from build123d import *

# Parameters (mm, degrees)
SKETCH1_W           = 23
SKETCH1_H           = 37.5
BOSS_EXTRUDE1_DEPTH = 48.5
SKETCH2_W           = 12.6
SKETCH2_H           = 24
CUT_EXTRUDE1_DEPTH  = 43.5
SKETCH3_W           = 12.6
SKETCH3_H           = 3
CUT_EXTRUDE2_DEPTH  = 5
SKETCH4_W           = 10
SKETCH4_H           = 2
BOSS_EXTRUDE2_DEPTH = 10
SKETCH5_W           = 10
SKETCH5_H           = 2
BOSS_EXTRUDE3_DEPTH = 10
SKETCH6_R           = 1.5
CUT_EXTRUDE3_DEPTH  = 10


with BuildPart() as part:
    # Sketch1 → Boss-Extrude1 (new body)
    with BuildSketch(Plane(origin=(0, 0, 0), x_dir=(1, 0, 0), z_dir=(0, 1, 0))):
        Rectangle(SKETCH1_W, SKETCH1_H)
    extrude(amount=BOSS_EXTRUDE1_DEPTH)

    # Sketch2 → Cut-Extrude1 (cut)
    with BuildSketch(Plane(origin=(0, 48.5, 0), x_dir=(1, 0, 0), z_dir=(0, 1, 0))):
        with Locations((0, -6.75)):
            Rectangle(SKETCH2_W, SKETCH2_H)
    extrude(amount=-CUT_EXTRUDE1_DEPTH, mode=Mode.SUBTRACT)

    # Sketch3 → Cut-Extrude2 (cut)
    with BuildSketch(Plane.XY.offset(-5.25)):
        with Locations((0, 26.5)):
            Rectangle(SKETCH3_W, SKETCH3_H)
    extrude(amount=-CUT_EXTRUDE2_DEPTH, mode=Mode.SUBTRACT)

    # Sketch4 → Boss-Extrude2 (add)
    with BuildSketch(Plane.ZY.offset(11.5)):
        with Locations((-13.75, 47.5)):
            Rectangle(SKETCH4_W, SKETCH4_H)
    extrude(amount=BOSS_EXTRUDE2_DEPTH)

    # Sketch5 → Boss-Extrude3 (add)
    with BuildSketch(Plane(origin=(11.5, 0, 0), x_dir=(0, 0, -1), z_dir=(1, 0, 0))):
        with Locations((13.75, 47.5)):
            Rectangle(SKETCH5_W, SKETCH5_H)
    extrude(amount=BOSS_EXTRUDE3_DEPTH)

    # Sketch6 → Cut-Extrude3 (cut)
    with BuildSketch(Plane(origin=(0, 48.5, 0), x_dir=(1, 0, 0), z_dir=(0, 1, 0))):
        with Locations(Location((16.5, 13.75, 0), (0, 0, 270))):
            Circle(SKETCH6_R)
        with Locations(Location((-16.5, 13.75, 0), (0, 0, 270))):
            Circle(SKETCH6_R)
    extrude(amount=-CUT_EXTRUDE3_DEPTH, mode=Mode.SUBTRACT)


solid = part.part
Model file for the job. Use its own axes, mm. A direction names the side the tool comes from. Coordinates: 2 decimals unless noted, no trailing zeros. Write each loop counter-clockwise with the first axis right and the second up, starting at its lowest first coordinate (ties: lowest second). Pieces come first, ordered by that corner, then holes. Notation, with made-up numbers: (-30.75, -11.75) - (23.25, -11.75) arc R14 ccw to (23.25, 1.25) - close; hole circle Ø9 at (15, -38.5). An arc over 180 degrees is marked (long way). Write each question's results on one line, items separated by ' | '. Start each with the question number.
1) 3-axis set-ups, long thin cutter, end or side, ignore diameter. For faces 5 (the face through (-15, 46.5, -15)), 6 (the face through (0, 5, 7)), 7 (the face through (0, 28, -8)): which of +Z, -Z, +X, -X, +Y, -Y reach the whole face in a straight line?
2) Cut at B-B (x = 16.5). Write the cut outline in (y, z), then the cut area to 3 significant figures.
3) Cut at D-D (x = 0). Write the cut outline in (y, z).
4) Cut at C-C (y = 32). Write the cut outline in (x, z), then the cut area to 3 significant figures.
5) Flat gauge pins, fed straight in: P1, Ø0.6, axis at x = 19, y = 47.5, coming from the +Z side; P2, Ø2.5, axis at x = -1.5, y = 27, coming from the +Z side; P3, Ø11, axis at x = -17.5, z = -12, coming from the -Y side; P4, Ø3, axis at x = -14, z = 1, coming from the -Y side. Where does each tip first touch, or does it go through?
6) Mould opens along Y. For faces 1 (the face through (0, 48.5, -8)), 2 (the face through (-16.43, 47.51, -15.25)), 3 (the face through (0, 27, -10.25)), 4 (the face through (15, 46.5, -13)) say: pulls with the +Y half, pulls with the -Y half, needs draft (parallel to the pull), parting line crosses it, or undercut.
7) Probe line 1 along X through (y, z) = (47.4, -13.75); line 2 along X through (y, z) = (42, 13); line 3 along X through (y, z) = (31, -17). List the from-to ranges inside material, lowest first. Write a range as from..to.
8) Cut at A-A (z = -13.75). Write the cut outline in (x, y), then the cut area to 3 significant figures.
Returned:
1) face 5: +Z, -Z, -X, -Y | face 6: +Z, +Y | face 7: +Z
2) outline: (46.5, -18.75) - (48.5, -18.75) - (48.5, -15.25) - (46.5, -15.25) - close; (46.5, -12.25) - (48.5, -12.25) - (48.5, -8.75) - (46.5, -8.75) - close | area: 14.0 mm^2
3) outline: (0, -18.75) - (48.5, -18.75) - (48.5, -5.25) - (28, -5.25) - (28, -10.25) - (25, -10.25) - (25, -5.25) - (5, -5.25) - (5, 18.75) - (0, 18.75) - close
4) outline: (-11.5, -18.75) - (11.5, -18.75) - (11.5, 18.75) - (6.3, 18.75) - (6.3, -5.25) - (-6.3, -5.25) - (-6.3, 18.75) - (-11.5, 18.75) - close | area: 560 mm^2
5) P1: z = -8.75 | P2: z = -5.25 | P3: y = 46.5 | P4: through
6) face 1: pulls with the +Y half | face 2: needs draft | face 3: undercut | face 4: pulls with the -Y half
7) line 1: -21.5..-18, -15..15, 18..21.5 | line 2: -11.5..-6.3, 6.3..11.5 | line 3: -11.5..11.5
8) outline: (-21.5, 46.5) - (-18, 46.5) - (-18, 48.5) - (-21.5, 48.5) - close; (-15, 46.5) - (-11.5, 46.5) - (-11.5, 0) - (11.5, 0) - (11.5, 46.5) - (15, 46.5) - (15, 48.5) - (-15, 48.5) - close; (18, 46.5) - (21.5, 46.5) - (21.5, 48.5) - (18, 48.5) - close | area: 1,140 mm^2
